Part model, mm, in its own coordinate system. A direction names the side the tool comes from. Round coordinates to 2 decimals unless told otherwise and drop trailing zeros. Loops run counter-clockwise (first coordinate to the right, second up) from the corner with the lowest first, then second, coordinate; pieces in that order, holes last.
1) Drop flat-ended pins along their axis: P1, Ø6, axis at x = 21.5, y = -54, coming from the +Z side; P2, Ø5, axis at x = 36.5, y = -4, coming from the -Z side. Give the stop position or say it passes through.
2) Band-saw the part on A-A, the plane y = -30. Write the cut outline in (x, z), then the cut area to 3 significant figures.
3) Probe line 1 (Y direction, x = 0, z = 4.75); line 2 (X direction, y = -30, z = 3); line 3 (Y direction, x = 50.5, z = 61). List the from-to ranges inside material, lowest first.
4) 3-axis set-ups, long thin cutter, end or side, ignore diameter. For faces 4 (the flat face through (55, -0.5, 9.5)), 5 (the flat face through (-1, -1, 10)): which of +Z, -Z, +X, -X, +Y, -Y reach the whole face in a straight line?
5) Mould opens along X. For faces 1 (the flat face through (-1, 100, 37)), 2 (the cylindrical face through (21.16, -31.69, 4.93)), 3 (the flat face through (-55, -0.5, 9.5)) say: +X half, -X half, draft (parallel to the pull), parting line (faces both ways), or undercut.
6) Band-saw the part on C-C, the plane x = 0. Write the cut outline in (y, z), then the cut area to 3 significant figures.
7) Band-saw the part on D-D, the plane z = 6.5. Write the cut outline in (x, y).
8) Band-saw the part on B-B, the plane z = 22.5. Write the cut outline in (x, y), then the cut area to 3 significant figures.
from build123d import *

# Parameters (mm, degrees)
SKETCH1_W           = 200
SKETCH1_H           = 110
BOSS_EXTRUDE1_DEPTH = 10
SKETCH2_W           = 110
SKETCH2_H           = 20
BOSS_EXTRUDE2_DEPTH = 65
SKETCH4_R           = 12.5
CUT_EXTRUDE1_DEPTH  = 76
SKETCH5_R           = 2.5
CUT_EXTRUDE2_DEPTH  = 76
SKETCH3_R           = 2.5
CUT_EXTRUDE3_DEPTH  = 76


with BuildPart() as part:
    # Sketch1 → Boss-Extrude1 (new body)
    with BuildSketch(Plane(origin=(0, 0, 0), x_dir=(0, 1, 0), z_dir=(0, 0, 1))):
        Rectangle(SKETCH1_W, SKETCH1_H)
    extrude(amount=BOSS_EXTRUDE1_DEPTH)

    # Sketch2 → Boss-Extrude2 (add)
    with BuildSketch(Plane.XY.offset(10)):
        with Locations((0, 90)):
            Rectangle(SKETCH2_W, SKETCH2_H)
        with Locations((0, -90)):
            Rectangle(SKETCH2_W, SKETCH2_H)
    extrude(amount=BOSS_EXTRUDE2_DEPTH)

    # Sketch4 → Cut-Extrude1 (cut, through all)
    with BuildSketch(Plane(origin=(0, 0, 0), x_dir=(1, 0, 0), z_dir=(0, 0, -1))):
        with Locations((0, 30)):
            Circle(SKETCH4_R)
    extrude(amount=-CUT_EXTRUDE1_DEPTH, mode=Mode.SUBTRACT)

    # Sketch5 → Cut-Extrude2 (cut, through all)
    with BuildSketch(Plane(origin=(0, 0, 0), x_dir=(1, 0, 0), z_dir=(0, 0, -1))):
        with Locations((23, 30)):
            Circle(SKETCH5_R)
        with Locations((-23, 30)):
            Circle(SKETCH5_R)
    extrude(amount=-CUT_EXTRUDE2_DEPTH, mode=Mode.SUBTRACT)

    # Sketch3 → Cut-Extrude3 (cut, through all)
    with BuildSketch(Plane(origin=(0, 0, 0), x_dir=(1, 0, 0), z_dir=(0, 0, -1))):
        with Locations((0, 55)):
            Circle(SKETCH3_R)
        with Locations((0, -15)):
            Circle(SKETCH3_R)
    extrude(amount=-CUT_EXTRUDE3_DEPTH, mode=Mode.SUBTRACT)


solid = part.part
Reported:
1. P1: stops at z = 10
1. P2: stops at z = 0
2. outline: (-55, 0) - (-25.5, 0) - (-25.5, 10) - (-55, 10) - close; (-20.5, 0) - (-12.5, 0) - (-12.5, 10) - (-20.5, 10) - close; (12.5, 0) - (20.5, 0) - (20.5, 10) - (12.5, 10) - close; (25.5, 0) - (55, 0) - (55, 10) - (25.5, 10) - close
2. area: 750 mm2
3. line 1: y = -100 to -57.5, -52.5 to -42.5, -17.5 to 12.5, 17.5 to 100
3. line 2: x = -55 to -25.5, -20.5 to -12.5, 12.5 to 20.5, 25.5 to 55
3. line 3: y = -100 to -80, 80 to 100
4. face 4: +Z, -Z, +X, +Y, -Y
4. face 5: +Z, +X, -X
5. face 1: draft
5. face 2: undercut
5. face 3: -X half
6. outline: (-100, 0) - (-57.5, 0) - (-57.5, 10) - (-80, 10) - (-80, 75) - (-100, 75) - close; (-52.5, 0) - (-42.5, 0) - (-42.5, 10) - (-52.5, 10) - close; (-17.5, 0) - (12.5, 0) - (12.5, 10) - (-17.5, 10) - close; (17.5, 0) - (100, 0) - (100, 75) - (80, 75) - (80, 10) - (17.5, 10) - close
6. area: 4,250 mm2
7. outline: (-55, -100) - (55, -100) - (55, 100) - (-55, 100) - close; hole circle Ø5 at (-23, -30); hole circle Ø25 at (0, -30); hole circle Ø5 at (0, -55); hole circle Ø5 at (0, 15); hole circle Ø5 at (23, -30)
8. outline: (-55, -100) - (55, -100) - (55, -80) - (-55, -80) - close; (-55, 80) - (55, 80) - (55, 100) - (-55, 100) - close
8. area: 4,400 mm2
